The listing builds one solid part. Answer for the finished solid, in the listing's coordinates (mm). Face numbers are marked on the shaded views. A direction names the side the tool comes from. Round coordinates to 2 decimals unless told otherwise and drop trailing zeros. Loops run counter-clockwise (first coordinate to the right, second up) from the corner with the lowest first, then second, coordinate; pieces in that order, holes last. Notation, with made-up numbers: (62, 22) -> (102, 22) arc R29 ccw to (102, 54) -> close; hole circle Ø9 at (86.5, -30). An arc over 180 degrees is marked (long way). Write each question's results on one line, items separated by ' | '. Start each with the question number.
(1) The part is cut by section C-C (z = 132.5). Determine the outline of the cut face in (x, y), plus the area to 3 significant figures.
(2) The part is cut by section B-B (y = 79). Determine the outline of the cut face in (x, z), plus the area to 3 significant figures.
(3) Straight lines are drawn through the part: probe 1 along X at (y, z) = (372.5, 128.5); probe 2 along X at (y, z) = (17.5, 424); probe 3 along Z at (x, y) = (57, 78). For each, find the intervals that lie inside material, in ascending order.
(4) Flat-ended cylindrical pins translate along their axes: pin 1 (13 mm diameter, centred on y = 353, z = 176.5, fed in from +X); pin 2 (12 mm diameter, centred on y = 315.5, z = 188, fed in from -X). Find the tip coordinate at first contact, or state that the pin passes through.
(5) Determine the mould class of the marked faces 3, 4, 5 and 6 for opening direction X: released by +X, released by -X, zero draft, split by the parting line, or undercut.
(6) The part is cut by section A-A (y = 173.5). Determine the outline of the cut face in (x, z).
(7) For the marked faces 1 and 2, determine the directions among +Z, -Z, +X, -X, +Y, -Y from which every point of the face is accessible in a straight line to the end or side of a thin tool.
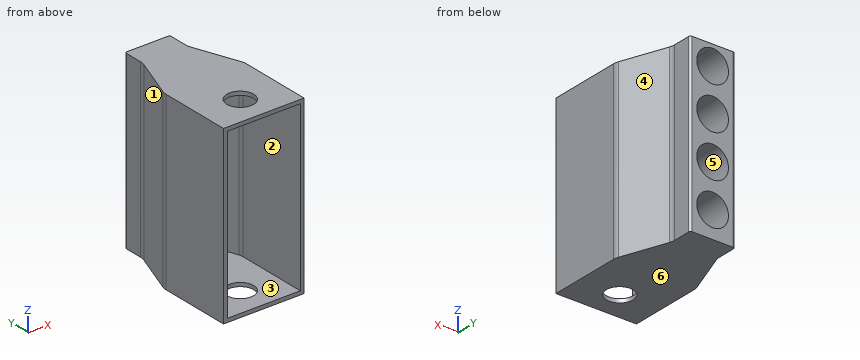
```python
from build123d import *

# Parameters (mm, degrees)
BOSS_EXTRUDE1_DEPTH  = 465
SHELL1_T             = -10
SKETCH3_R            = 36
CUT_EXTRUDE2_DEPTH   = 570
SKETCH2_R            = 42.5
CUT_EXTRUDE3_DEPTH   = 10
SKETCH6_R            = 45.5
SKETCH6_R_2          = 42.5
BOSS_EXTRUDE14_DEPTH = 120


with BuildPart() as part:
    # Sketch1 → Boss-Extrude1 (new body)
    with BuildSketch(Plane.XY):
        with BuildLine():
            Line((107.802304208, 0), (-107.802304208, 0))
            Line((-107.802304208, 0), (-107.802304208, 192.946920772))
            ThreePointArc((-107.802304208, 192.946920772), (-107.194614328, 199.892847878), (-105.390009039, 206.627726505))
            Line((-105.390009039, 206.627726505), (-62.412295169, 324.708024904))
            ThreePointArc((-62.412295169, 324.708024904), (-60.60768988, 331.442903531), (-60, 338.388830637))
            Line((-60, 338.388830637), (-60, 386))
            ThreePointArc((-60, 386), (-58.535533906, 389.535533906), (-55, 391))
            Line((-55, 391), (55, 391))
            ThreePointArc((55, 391), (58.535533906, 389.535533906), (60, 386))
            Line((60, 386), (60, 338.388830637))
            ThreePointArc((60, 338.388830637), (60.60768988, 331.442903531), (62.412295169, 324.708024904))
            Line((62.412295169, 324.708024904), (105.390009039, 206.627726505))
            ThreePointArc((105.390009039, 206.627726505), (107.194614328, 199.892847878), (107.802304208, 192.946920772))
            Line((107.802304208, 192.946920772), (107.802304208, 0))
        make_face()
    extrude(amount=BOSS_EXTRUDE1_DEPTH)

    # Shell1
    shell1_openings = [part.faces().sort_by_distance(p)[0] for p in [
        (0, 0, 232.5),
    ]]
    offset(amount=SHELL1_T, openings=shell1_openings, kind=Kind.INTERSECTION)

    # Sketch3 → Cut-Extrude2 (cut)
    with BuildSketch(Plane.XY.offset(465)):
        with Locations(Location((0, 79, 0), (0, 0, 180))):
            Circle(SKETCH3_R)
    extrude(amount=-CUT_EXTRUDE2_DEPTH, mode=Mode.SUBTRACT)

    # Sketch2 → Cut-Extrude3 (cut)
    with BuildSketch(Plane(origin=(0, 391, 0), x_dir=(1, 0, 0), z_dir=(0, 1, 0))):
        with Locations(Location((0, -70.502440314, 0), (0, 0, 270))):
            Circle(SKETCH2_R)
        with Locations(Location((0, -184.502440314, 0), (0, 0, 270))):
            Circle(SKETCH2_R)
        with Locations(Location((0, -298.502440314, 0), (0, 0, 270))):
            Circle(SKETCH2_R)
        with Locations(Location((0, -412.502440314, 0), (0, 0, 270))):
            Circle(SKETCH2_R)
    extrude(amount=-CUT_EXTRUDE3_DEPTH, mode=Mode.SUBTRACT)

    # Sketch6 → Boss-Extrude14 (add)
    # profile 1 of 4: a face of its own
    with BuildSketch(Plane(origin=(0, 391, 0), x_dir=(1, 0, 0), z_dir=(0, 1, 0))):
        with Locations((0, -412.502440314)):
            Circle(SKETCH6_R)
        with Locations(Location((0, -412.502440314, 0), (0, 0, 270))):
            Circle(SKETCH6_R_2, mode=Mode.SUBTRACT)
    # profile 2 of 4: a face of its own
    with BuildSketch(Plane(origin=(0, 391, 0), x_dir=(1, 0, 0), z_dir=(0, 1, 0))):
        with Locations(Location((0, -298.502440314, 0), (0, 0, 270))):
            Circle(SKETCH6_R)
        with Locations(Location((0, -298.502440314, 0), (0, 0, 270))):
            Circle(SKETCH6_R_2, mode=Mode.SUBTRACT)
    # profile 3 of 4: a face of its own
    with BuildSketch(Plane(origin=(0, 391, 0), x_dir=(1, 0, 0), z_dir=(0, 1, 0))):
        with Locations(Location((0, -184.502440314, 0), (0, 0, 270))):
            Circle(SKETCH6_R)
        with Locations(Location((0, -184.502440314, 0), (0, 0, 270))):
            Circle(SKETCH6_R_2, mode=Mode.SUBTRACT)
    # profile 4 of 4: a face of its own
    with BuildSketch(Plane(origin=(0, 391, 0), x_dir=(1, 0, 0), z_dir=(0, 1, 0))):
        with Locations(Location((0, -70.502440314, 0), (0, 0, 270))):
            Circle(SKETCH6_R)
        with Locations(Location((0, -70.502440314, 0), (0, 0, 270))):
            Circle(SKETCH6_R_2, mode=Mode.SUBTRACT)
    extrude(amount=-BOSS_EXTRUDE14_DEPTH)


solid = part.part
```
Checked values:
1) outline: (-107.8, 0) -> (-97.8, 0) -> (-97.8, 192.95) arc R30 cw to (-95.99, 203.21) -> (-53.02, 321.29) arc R50 ccw to (-50, 338.39) -> (-50, 381) -> (50, 381) -> (50, 338.39) arc R50 ccw to (53.02, 321.29) -> (95.99, 203.21) arc R30 cw to (97.8, 192.95) -> (97.8, 0) -> (107.8, 0) -> (107.8, 192.95) arc R40 ccw to (105.39, 206.63) -> (62.41, 324.71) arc R40 cw to (60, 338.39) -> (60, 386) arc R5 ccw to (55, 391) -> (-55, 391) arc R5 ccw to (-60, 386) -> (-60, 338.39) arc R40 cw to (-62.41, 324.71) -> (-105.39, 206.63) arc R40 ccw to (-107.8, 192.95) -> close | area: 8,970 mm2
2) outline: (-107.8, 0) -> (-36, 0) -> (-36, 10) -> (-97.8, 10) -> (-97.8, 455) -> (-36, 455) -> (-36, 465) -> (-107.8, 465) -> close; (36, 0) -> (107.8, 0) -> (107.8, 465) -> (36, 465) -> (36, 455) -> (97.8, 455) -> (97.8, 10) -> (36, 10) -> close | area: 11,800 mm2
3) probe 1: x = -60 to -50, 50 to 60 | probe 2: x = -107.8 to -97.8, 97.8 to 107.8 | probe 3: z = 0 to 10, 455 to 465
4) pin 1: stops at x = 60 | pin 2: stops at x = -67.95
5) face 3: undercut | face 4: released by +X | face 5: undercut | face 6: zero draft
6) outline: (-107.8, 0) -> (107.8, 0) -> (107.8, 465) -> (-107.8, 465) -> close; hole (-97.8, 10) -> (97.8, 10) -> (97.8, 455) -> (-97.8, 455) -> close
7) face 1: +Z, -Z, -X, +Y | face 2: -Y
